from build123d import *

# Parameters (mm, degrees)
EXTRUDE_1_DEPTH     = 3
SKETCH_2_W          = 53
SKETCH_2_H          = 28
EXTRUDE_2_DEPTH     = 3
SKETCH_3_R          = 2
CUT_EXTRUDE_1_DEPTH = 157.901242825


with BuildPart() as part:
    # 草图1 → 凸台-拉伸1 (new body)
    with BuildSketch(Plane(origin=(0, 0, 0), x_dir=(1, 0, 0), z_dir=(0, 1, 0))):
        with BuildLine():
            Line((117, 0), (142, 0))
            Line((142, 0), (142, 53))
            Line((142, 53), (117, 53))
            ThreePointArc((117, 53), (112.16726189, 41.33273811), (100.5, 36.5))
            Line((100.5, 36.5), (0, 36.5))
            Line((0, 36.5), (0, 16.5))
            Line((0, 16.5), (100.5, 16.5))
            ThreePointArc((100.5, 16.5), (112.16726189, 11.66726189), (117, 0))
        make_face()
    extrude(amount=EXTRUDE_1_DEPTH)

    # 草图2 → 凸台-拉伸2 (add)
    with BuildSketch(Plane(origin=(142, 0, 0), x_dir=(0, 0, -1), z_dir=(1, 0, 0))):
        with Locations((26.5, 14)):
            Rectangle(SKETCH_2_W, SKETCH_2_H)
    extrude(amount=EXTRUDE_2_DEPTH)

    # 草图3 → 切除-拉伸1 (cut, through all)
    with BuildSketch(Plane(origin=(145, 0, 0), x_dir=(0, 0, -1), z_dir=(1, 0, 0))):
        with Locations((50, 23.5)):
            Circle(SKETCH_3_R)
        with Locations(Location((3, 23.5, 0), (0, 0, 180))):
            Circle(SKETCH_3_R)
    extrude(amount=-CUT_EXTRUDE_1_DEPTH, mode=Mode.SUBTRACT)


solid = part.part
Can you work these out from the model? Positions are in its coordinate system, mm. A direction names the side the tool comes from. Give positions to 0.01 mm unless a question says otherwise; leave off trailing zeros. Order: outer loops, then holes, each group sorted by start corner. A loop starts at its lowest first (then second) coordinate and runs counter-clockwise, first axis right, second up. Notation, with made-up numbers: M 54.5,48.5 L 89.5,48.5 A30 ccw 89.5,79.5 Z; hole C -23.5,-33.75 d7. An arc over 180 degrees is marked long. Use one line per item in the form item = value.
Item 1: Will these pins go through, and if not, where does the flat tip stop? pin 1 Ø10 at (y, z) = (6.5, -43) entering from -X; pin 2 Ø5 at (x, z) = (102, -26) entering from +Y; pin 3 Ø6 at (x, z) = (44.5, -35) entering from -Y; pin 4 Ø2 at (x, y) = (74.5, 5.5) entering from -Z.
Values follow:
pin_1 = 109.89
pin_2 = 3
pin_3 = 0
pin_4 = through
Item 2: If I drill on line 1 along Y through (x, z) = (142.75, -50); line 2 along X through (y, z) = (19, -9.5); line 3 along Y through (x, z) = (65.5, -23.5), over which ranges is the centre line in solid material (lowest first)? Write a range as [from, to].
Values follow:
line_1 = [0, 21.5], [25.5, 28]
line_2 = [142, 145]
line_3 = [0, 3]
Item 3: If we section it at D-D, the plane x = 72.5: Write out the boundary of the cut face in (y, z).
Values follow:
outline = M 0,-36.5 L 3,-36.5 L 3,-16.5 L 0,-16.5 Z
Item 4: Thinking about a two-plate mould opening in Y: for faces 6 (the cylindrical face through (143.521, 22.734, -51.847)), 7 (the flat face through (145, 14, -26)), 8 (the flat face through (143, 28, -26)), which applies, pulls with the +Y half, pulls with the -Y half, needs draft (parallel to the pull), parting line crosses it, or undercut?
Values follow:
face_6 = undercut
face_7 = needs draft
face_8 = pulls with the +Y half
Item 5: If we section it at B-B, the plane z = -21: Write out the boundary of the cut face in (x, y), and give its area (3 significant figures).
Values follow:
outline = M 0,0 L 145,0 L 145,28 L 142,28 L 142,3 L 0,3 Z
area = 510 mm^2
Item 6: If we section it at A-A, the plane y = 23.5: Write out the boundary of the cut face in (x, z), and give its area (3 significant figures).
Values follow:
outline = M 142,-53 L 145,-53 L 145,-52 L 142,-52 Z; M 142,-48 L 145,-48 L 145,-5 L 142,-5 Z; M 142,-1 L 145,-1 L 145,0 L 142,0 Z
area = 135 mm^2
Item 7: If we section it at C-C, the plane z = -50: Write out the boundary of the cut face in (x, y).
Values follow:
outline = M 116.72,0 L 145,0 L 145,21.5 L 142,21.5 L 142,3 L 116.72,3 Z; M 142,25.5 L 145,25.5 L 145,28 L 142,28 Z
Item 8: For faces 1 (the flat face through (0, 1, -27)), 2 (the flat face through (86, 3, -27)), 3 (the flat face through (88, 0, -26)), 4 (the flat face through (50, 1, -16.5)), 5 (the flat face through (51, 1, -36.5)), which set-ups out of +Z, -Z, +X, -X, +Y, -Y let a thin tool reach every point of the face, with its end or its side?
Values follow:
face_1 = +Z, -Z, -X, +Y, -Y
face_2 = +Z, -Z, -X, +Y
face_3 = +Z, -Z, +X, -X, -Y
face_4 = +Z, -X, +Y, -Y
face_5 = -Z, -X, +Y, -Y
